Read the model definition and answer for the solid it produces. Units are mm, in the model's axes. Face numbers are marked on the shaded views. A direction names the side the tool comes from. Give positions to 0.01 mm unless a question says otherwise; leave off trailing zeros. Order: outer loops, then holes, each group sorted by start corner. A loop starts at its lowest first (then second) coordinate and runs counter-clockwise, first axis right, second up.
Item 1: A cutting plane is placed at D-D (x = -9). Write down the section's boundary in (y, z).
Item 2: Which of the six approach directions +Z, -Z, +X, -X, +Y, -Y give full straight-line access (tool end or side, diameter ignored) to the marked faces 4, 5 and 6?
Item 3: A cutting plane is placed at A-A (z = -16.5). Write down the section's boundary in (x, y), plus the area to 3 significant figures.
Item 4: A cutting plane is placed at C-C (x = -25). Write down the section's boundary in (y, z).
Item 5: A cutting plane is placed at B-B (x = 19). Write down the section's boundary in (y, z), plus the area to 3 significant figures.
Item 6: The mould has two halves that part along X. Classify the marked faces 1, 2 and 3: +X half, -X half, draft (parallel to the pull), parting line (faces both ways), or undercut.
Item 7: Given pin 1 Ø6.5 at (y, z) = (17.5, -31) entering from -X; pin 2 Ø14 at (x, y) = (3, 14) entering from +Z; pin 3 Ø10 at (y, z) = (14.5, 30.5) entering from +X; pin 4 Ø4 at (x, z) = (19.5, 17) entering from +Y, each flat-ended and moving along its own axis, determine where each tip first touches the part or whether it passes through.
Item 8: Find the intervals of material crossed by line 1 along X through (y, z) = (21, -10); line 2 along X through (y, z) = (19, 27.5), in increasing order.
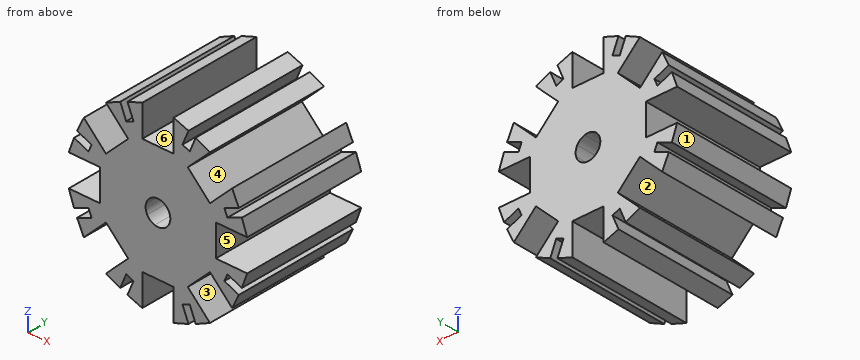
from build123d import *

# Parameters (mm, degrees)
BOSS_EXTRUDE3_DEPTH = 50.8
CIRPATTERN2_COUNT   = 8


with BuildPart() as part:
    # Sketch1 → Boss-Extrude3 (new body)
    with BuildSketch(Plane(origin=(0, 0, 0), x_dir=(1, 0, 0), z_dir=(0, 1, 0))):
        with BuildLine():
            Line((21.052414425, 12.072158304), (12.072158304, 21.052414425))
            Line((12.072158304, 21.052414425), (2.487247326, 4.337464782))
            ThreePointArc((2.487247326, 4.337464782), (3.957792808, 3.055466591), (4.825800212, 1.30830131))
            Line((4.825800212, 1.30830131), (23.42261, 6.35))
            Line((23.42261, 6.35), (36.12261, 6.35))
            Line((36.12261, 6.35), (33.980449989, 12.356865623))
            Line((33.980449989, 12.356865623), (28.113814957, 9.926825827))
            Line((28.113814957, 9.926825827), (26.89879506, 12.860143343))
            Line((26.89879506, 12.860143343), (32.765430091, 15.290183139))
            Line((32.765430091, 15.290183139), (30.032670546, 21.052414425))
            Line((30.032670546, 21.052414425), (21.052414425, 12.072158304))
        make_face()
    extrude(amount=BOSS_EXTRUDE3_DEPTH)


with BuildPart() as cirpattern2_1:
    # CirPattern2: pattern copy
    add(part.part.rotate(Axis((0, 0, 0), (0, 1, 0)), 1 * 360 / CIRPATTERN2_COUNT))


with BuildPart() as cirpattern2_2:
    # CirPattern2: pattern copy
    add(part.part.rotate(Axis((0, 0, 0), (0, 1, 0)), 2 * 360 / CIRPATTERN2_COUNT))


with BuildPart() as cirpattern2_3:
    # CirPattern2: pattern copy
    add(part.part.rotate(Axis((0, 0, 0), (0, 1, 0)), 3 * 360 / CIRPATTERN2_COUNT))


with BuildPart() as cirpattern2_4:
    # CirPattern2: pattern copy
    add(part.part.rotate(Axis((0, 0, 0), (0, 1, 0)), 4 * 360 / CIRPATTERN2_COUNT))


with BuildPart() as cirpattern2_5:
    # CirPattern2: pattern copy
    add(part.part.rotate(Axis((0, 0, 0), (0, 1, 0)), 5 * 360 / CIRPATTERN2_COUNT))


with BuildPart() as cirpattern2_6:
    # CirPattern2: pattern copy
    add(part.part.rotate(Axis((0, 0, 0), (0, 1, 0)), 6 * 360 / CIRPATTERN2_COUNT))


with BuildPart() as cirpattern2_7:
    # CirPattern2: pattern copy
    add(part.part.rotate(Axis((0, 0, 0), (0, 1, 0)), 7 * 360 / CIRPATTERN2_COUNT))


with BuildPart() as cirpattern2_1_1:
    add(cirpattern2_1.part)

    # Combine2: union CirPattern2_2, CirPattern2_3, CirPattern2_4, CirPattern2_5, CirPattern2_6, CirPattern2_7, part
    add(cirpattern2_2.part)
    add(cirpattern2_3.part)
    add(cirpattern2_4.part)
    add(cirpattern2_5.part)
    add(cirpattern2_6.part)
    add(cirpattern2_7.part)
    add(part.part)


solid = cirpattern2_1_1.part
Response values:
1. outline: (0, -35.18) - (50.8, -35.18) - (50.8, 35.18) - (0, 35.18) - close
2. face 4: +Y, -Y
2. face 5: +X, +Y, -Y
2. face 6: +Z, +Y, -Y
3. outline: (-32.19, 0) - (-25.48, 0) - (-25.48, 50.8) - (-32.19, 50.8) - close; (-16.62, 0) - (16.62, 0) - (16.62, 50.8) - (-16.62, 50.8) - close; (25.48, 0) - (32.19, 0) - (32.19, 50.8) - (25.48, 50.8) - close
3. area: 2,370 mm2
4. outline: (0, -16.02) - (50.8, -16.02) - (50.8, -6.35) - (0, -6.35) - close; (0, 6.35) - (50.8, 6.35) - (50.8, 16.02) - (0, 16.02) - close
5. outline: (0, -31.01) - (50.8, -31.01) - (50.8, -27.98) - (0, -27.98) - close; (0, -14.12) - (50.8, -14.12) - (50.8, 14.12) - (0, 14.12) - close; (0, 27.98) - (50.8, 27.98) - (50.8, 31.01) - (0, 31.01) - close
5. area: 1,740 mm2
6. face 1: -X half
6. face 2: undercut
6. face 3: +X half
7. pin 1: stops at x = -21.05
7. pin 2: stops at z = 36.12
7. pin 3: stops at x = 21.05
7. pin 4: passes through
8. line 1: x = -34.82 to -28.29, -28.08 to 28.08, 28.29 to 34.82
8. line 2: x = -18.52 to -13.11, -11.41 to -6.35, 6.35 to 11.41, 13.11 to 18.52
